For this review, take the finished solid that the model builds, in its own axes (mm). A direction names the side the tool comes from. Give positions to 0.01 mm unless a question says otherwise; leave off trailing zeros. Write each loop counter-clockwise with the first axis right and the second up, starting at its lowest first coordinate (ties: lowest second). Pieces come first, ordered by that corner, then holes. Notation, with made-up numbers: (14.25, 52.5) -> (22.25, 52.5) arc R24 cw to (22.25, 67.5) -> close; hole circle Ø3 at (-2, -22.75). An arc over 180 degrees is marked (long way). Return JSON: item names as keys, results as strings.
from build123d import *

# Parameters (mm, degrees)
BOSS_EXTRUDE1_DEPTH = 6.35


with BuildPart() as part:
    # Sketch1 → Boss-Extrude1 (new body)
    with BuildSketch(Plane(origin=(0, 0, 0), x_dir=(1, 0, 0), z_dir=(0, 1, 0))):
        with BuildLine():
            Line((-85.499768134, 67.575454856), (-53.631298012, 67.575454856))
            Line((-53.631298012, 67.575454856), (-53.631298012, 64.400454856))
            Line((-53.631298012, 64.400454856), (-55.383898012, 64.400454856))
            Line((-55.383898012, 64.400454856), (-55.383898012, 61.860454856))
            Line((-55.383898012, 61.860454856), (-53.631298012, 61.860454856))
            Line((-53.631298012, 61.860454856), (-53.631298012, 60.590454856))
            Line((-53.631298012, 60.590454856), (-50.583438656, 60.590454856))
            Line((-50.583438656, 60.590454856), (-50.583438656, 61.860454856))
            Line((-50.583438656, 61.860454856), (-48.830838656, 61.860454856))
            Line((-48.830838656, 61.860454856), (-48.830838656, 64.400454856))
            Line((-48.830838656, 64.400454856), (-50.583438656, 64.400454856))
            Line((-50.583438656, 64.400454856), (-50.583438656, 67.575454856))
            Line((-50.583438656, 67.575454856), (-17.182368334, 67.575454856))
            Line((-17.182368334, 67.575454856), (-17.182368334, 73.925454856))
            Line((-17.182368334, 73.925454856), (8.217631666, 73.925454856))
            Line((8.217631666, 73.925454856), (8.217631666, 67.575454856))
            Line((8.217631666, 67.575454856), (41.618701988, 67.575454856))
            Line((41.618701988, 67.575454856), (41.618701988, 64.400454856))
            Line((41.618701988, 64.400454856), (39.866101988, 64.400454856))
            Line((39.866101988, 64.400454856), (39.866101988, 61.860454856))
            Line((39.866101988, 61.860454856), (41.618701988, 61.860454856))
            Line((41.618701988, 61.860454856), (41.618701988, 60.590454856))
            Line((41.618701988, 60.590454856), (44.666561344, 60.590454856))
            Line((44.666561344, 60.590454856), (44.666561344, 61.860454856))
            Line((44.666561344, 61.860454856), (46.419161344, 61.860454856))
            Line((46.419161344, 61.860454856), (46.419161344, 64.400454856))
            Line((46.419161344, 64.400454856), (44.666561344, 64.400454856))
            Line((44.666561344, 64.400454856), (44.666561344, 67.575454856))
            Line((44.666561344, 67.575454856), (79.600231866, 67.575454856))
            ThreePointArc((79.600231866, 67.575454856), (88.580487987, 63.855710977), (92.300231866, 54.875454856))
            Line((92.300231866, 54.875454856), (92.306789937, 37.730454856))
            Line((92.306789937, 37.730454856), (85.971363429, 37.730454856))
            Line((85.971363429, 37.730454856), (85.971363429, -38.469545144))
            Line((85.971363429, -38.469545144), (92.321363429, -38.469545144))
            Line((92.321363429, -38.469545144), (92.342494993, -55.614545144))
            ThreePointArc((92.342494993, -55.614545144), (88.622751114, -64.594801265), (79.642494993, -68.314545144))
            Line((79.642494993, -68.314545144), (44.666561344, -68.314545144))
            Line((44.666561344, -68.314545144), (44.666561344, -65.139545144))
            Line((44.666561344, -65.139545144), (46.419161344, -65.139545144))
            Line((46.419161344, -65.139545144), (46.419161344, -62.599545144))
            Line((46.419161344, -62.599545144), (44.666561344, -62.599545144))
            Line((44.666561344, -62.599545144), (44.666561344, -61.329545144))
            Line((44.666561344, -61.329545144), (41.618701988, -61.329545144))
            Line((41.618701988, -61.329545144), (41.618701988, -62.599545144))
            Line((41.618701988, -62.599545144), (39.866101988, -62.599545144))
            Line((39.866101988, -62.599545144), (39.866101988, -65.139545144))
            Line((39.866101988, -65.139545144), (41.618701988, -65.139545144))
            Line((41.618701988, -65.139545144), (41.618701988, -68.314545144))
            Line((41.618701988, -68.314545144), (8.217631666, -68.314545144))
            Line((8.217631666, -68.314545144), (8.217631666, -74.664545144))
            Line((8.217631666, -74.664545144), (-17.182368334, -74.664545144))
            Line((-17.182368334, -74.664545144), (-17.182368334, -68.314545144))
            Line((-17.182368334, -68.314545144), (-50.583438656, -68.314545144))
            Line((-50.583438656, -68.314545144), (-50.583438656, -65.139545144))
            Line((-50.583438656, -65.139545144), (-48.830838656, -65.139545144))
            Line((-48.830838656, -65.139545144), (-48.830838656, -62.599545144))
            Line((-48.830838656, -62.599545144), (-50.583438656, -62.599545144))
            Line((-50.583438656, -62.599545144), (-50.583438656, -61.329545144))
            Line((-50.583438656, -61.329545144), (-53.631298012, -61.329545144))
            Line((-53.631298012, -61.329545144), (-53.631298012, -62.599545144))
            Line((-53.631298012, -62.599545144), (-55.383898012, -62.599545144))
            Line((-55.383898012, -62.599545144), (-55.383898012, -65.139545144))
            Line((-55.383898012, -65.139545144), (-53.631298012, -65.139545144))
            Line((-53.631298012, -65.139545144), (-53.631298012, -68.314545144))
            Line((-53.631298012, -68.314545144), (-85.499768134, -68.314545144))
            Line((-85.499768134, -68.314545144), (-85.499768134, -52.693474822))
            Line((-85.499768134, -52.693474822), (-82.324768134, -52.693474822))
            Line((-82.324768134, -52.693474822), (-82.324768134, -54.446074822))
            Line((-82.324768134, -54.446074822), (-79.784768134, -54.446074822))
            Line((-79.784768134, -54.446074822), (-79.784768134, -52.693474822))
            Line((-79.784768134, -52.693474822), (-78.514768134, -52.693474822))
            Line((-78.514768134, -52.693474822), (-78.514768134, -49.645615466))
            Line((-78.514768134, -49.645615466), (-79.784768134, -49.645615466))
            Line((-79.784768134, -49.645615466), (-79.784768134, -47.893015466))
            Line((-79.784768134, -47.893015466), (-82.324768134, -47.893015466))
            Line((-82.324768134, -47.893015466), (-82.324768134, -49.645615466))
            Line((-82.324768134, -49.645615466), (-85.499768134, -49.645615466))
            Line((-85.499768134, -49.645615466), (-85.499768134, -38.469545144))
            Line((-85.499768134, -38.469545144), (-91.849768134, -38.469545144))
            Line((-91.849768134, -38.469545144), (-91.849768134, -13.069545144))
            Line((-91.849768134, -13.069545144), (-85.499768134, -13.069545144))
            Line((-85.499768134, -13.069545144), (-85.499768134, -1.893474822))
            Line((-85.499768134, -1.893474822), (-82.324768134, -1.893474822))
            Line((-82.324768134, -1.893474822), (-82.324768134, -3.646074822))
            Line((-82.324768134, -3.646074822), (-79.784768134, -3.646074822))
            Line((-79.784768134, -3.646074822), (-79.784768134, -1.893474822))
            Line((-79.784768134, -1.893474822), (-78.514768134, -1.893474822))
            Line((-78.514768134, -1.893474822), (-78.514768134, 1.154384534))
            Line((-78.514768134, 1.154384534), (-79.784768134, 1.154384534))
            Line((-79.784768134, 1.154384534), (-79.784768134, 2.906984534))
            Line((-79.784768134, 2.906984534), (-82.324768134, 2.906984534))
            Line((-82.324768134, 2.906984534), (-82.324768134, 1.154384534))
            Line((-82.324768134, 1.154384534), (-85.499768134, 1.154384534))
            Line((-85.499768134, 1.154384534), (-85.499768134, 12.330454856))
            Line((-85.499768134, 12.330454856), (-91.849768134, 12.330454856))
            Line((-91.849768134, 12.330454856), (-91.849768134, 37.730454856))
            Line((-91.849768134, 37.730454856), (-85.499768134, 37.730454856))
            Line((-85.499768134, 37.730454856), (-85.499768134, 48.906525178))
            Line((-85.499768134, 48.906525178), (-82.324768134, 48.906525178))
            Line((-82.324768134, 48.906525178), (-82.324768134, 47.153925178))
            Line((-82.324768134, 47.153925178), (-79.784768134, 47.153925178))
            Line((-79.784768134, 47.153925178), (-79.784768134, 48.906525178))
            Line((-79.784768134, 48.906525178), (-78.514768134, 48.906525178))
            Line((-78.514768134, 48.906525178), (-78.514768134, 51.954384534))
            Line((-78.514768134, 51.954384534), (-79.784768134, 51.954384534))
            Line((-79.784768134, 51.954384534), (-79.784768134, 53.706984534))
            Line((-79.784768134, 53.706984534), (-82.324768134, 53.706984534))
            Line((-82.324768134, 53.706984534), (-82.324768134, 51.954384534))
            Line((-82.324768134, 51.954384534), (-85.499768134, 51.954384534))
            Line((-85.499768134, 51.954384534), (-85.499768134, 67.575454856))
        make_face()
    extrude(amount=BOSS_EXTRUDE1_DEPTH)


solid = part.part
1. To check wall thickness, follow probe 1 along Z at (x, y) = (40, 4); probe 2 along X at (y, z) = (3.75, 62); probe 3 along X at (y, z) = (4.75, 9). State the ranges of each line that lie inside material, in increasing order.
Results found:
{"probe 1": "z = -67.58 to -64.4, -61.86 to 62.6, 65.14 to 68.31", "probe 2": "x = -85.5 to -53.63, -50.58 to 41.62, 44.67 to 90.62", "probe 3": "x = -85.5 to 85.97"}
2. Add section B-B, the plane x = -33. State the section outline as (y, z) points, plus the area to 3 significant figures.
Results found:
{"outline": "(0, -67.58) -> (6.35, -67.58) -> (6.35, 68.31) -> (0, 68.31) -> close", "area": "863 mm²"}
3. The part is to be moulded in two halves that separate along Z. For faces 1 (the flat face through (-89, 3, -37.73)), 2 (the flat face through (-91.85, 3, 26)), 3 (the flat face through (-89, 3, 13.07)), 4 (the flat face through (62, 3, 68.315)), say which applies: +Z half, -Z half, draft (parallel to the pull), parting line (faces both ways), or undercut.
Results found:
{"face 1": "-Z half", "face 2": "draft", "face 3": "undercut", "face 4": "+Z half"}
4. For faces 5 (the flat face through (-91.85, 3, -25)), 6 (the flat face through (-17.182, 3, -71)), 7 (the flat face through (25, 3, -67.575)), 8 (the flat face through (-69, 3, 68.315)), list the 3-axis set-ups (+Z, -Z, +X, -X, +Y, -Y) from which the entire face can be reached by the end or side of a thin tool; tool diameter is ignored.
Results found:
{"face 5": "+Z, -Z, -X, +Y, -Y", "face 6": "-Z, -X, +Y, -Y", "face 7": "-Z, +X, +Y, -Y", "face 8": "+Z, -X, +Y, -Y"}
5. Add section A-A, the plane z = 10.5. State the section outline as (x, y) points, plus the area to 3 significant figures.
Results found:
{"outline": "(-85.5, 0) -> (85.97, 0) -> (85.97, 6.35) -> (-85.5, 6.35) -> close", "area": "1,090 mm²"}
6. For pin 1 (3 mm diameter, centred on y = 5, z = -51.5, fed in from -X); pin 2 (1.6 mm diameter, centred on y = 2.5, z = -65, fed in from +X); pin 3 (0.9 mm diameter, centred on y = 2.5, z = -48, fed in from +X), all flat-tipped, find the tip position at first contact; note any pin that passes through.
Results found:
{"pin 1": "stops at x = -85.5", "pin 2": "stops at x = 88.22", "pin 3": "stops at x = 92.3"}
